Autodesk Inventor part; units mm, degrees
ref_plane "YZ Plane" through (0, 0, 0) normal (1, 0, 0) x (0, 1, 0)
ref_plane "XZ Plane" through (0, 0, 0) normal (0, 1, 0) x (-1, 0, 0)
ref_plane "XY Plane" through (0, 0, 0) normal (0, 0, 1) x (1, 0, 0)
sketch "草图1" plane through (0, 0, 0) normal (0, 0, 1) x (1, 0, 0)
  circle A0 centre (0, 0) radius 2.5
  dimension "d0" = 5
extrude "拉伸1" add sketch "草图1" along normal blind 3
sketch "草图2" plane through (0, 0, 3) normal (0, 0, 1) x (1, 0, 0)
  line L0 (-0.75, 2.5) -> (0.75, 2.5)
  line L1 (0.75, 2.5) -> (0.75, -2.5)
  line L2 (0.75, -2.5) -> (-0.75, -2.5)
  line L3 (-0.75, -2.5) -> (-0.75, 2.5)
  circle A0 centre (0, 0) radius 2.5
  point P0 (0, 2.5)
  dimension "d3" = 1.5
extrude "拉伸2" cut sketch "草图2" against normal blind 1.5 contours L0 A0 L3 | L0 L1 A0 | A0 L1 L3 | A0 L2 L3 | L1 L2 A0
sketch "草图3" plane through (0, 0, 0) normal (0, 0, -1) x (-1, 0, 0)
  circle A0 centre (0, 0) radius 1.5
  dimension "d6" = 3
extrude "拉伸3" add sketch "草图3" along normal blind 10
thread "螺纹1"
chamfer "倒角1" distance 0.2 angle 45 1 edges at (1.5, 0, -10)
properties part number "分离前导形片固定螺丝"
Work out the finished part from the listing and answer in its coordinate system (mm). A direction names the side the tool comes from. Give positions to 0.01 mm unless a question says otherwise; leave off trailing zeros. Loops run counter-clockwise (first coordinate to the right, second up) from the corner with the lowest first, then second, coordinate; pieces in that order, holes last. Notation, with made-up numbers: (25.25, -25.75) - (82.25, -25.75) arc R30 ccw to (82.25, 11.25) - close; hole circle Ø5 at (-38, -25.5). An arc over 180 degrees is marked (long way). Answer in a Markdown table with one row per item.
(1) Section C-C (z = 0.25) is taken. Give the vertices of the cut face in (x, y), and give its area (3 significant figures).
Results list:
| item | result |
|---|---|
| outline | circle Ø5 at (0, 0) |
| area | 19.6 mm² |
(2) Section D-D (y = -1.65) is taken. Give the vertices of the cut face in (x, z).
Results list:
| item | result |
|---|---|
| outline | (-1.88, 0) - (1.88, 0) - (1.88, 3) - (0.75, 3) - (0.75, 1.5) - (-0.75, 1.5) - (-0.75, 3) - (-1.88, 3) - close |
(3) Consider L1, parallel to Z at x = 2.15, y = -0.9; L2, parallel to Y at x = 0, z = -1.5; L3, parallel to Z at x = -0.4, y = -1.85. Determine where each line is inside the solid, lowest interval first. Write a range as [from, to].
Results list:
| item | result |
|---|---|
| L1 | z = [0, 3] |
| L2 | y = [-1.5, 1.5] |
| L3 | z = [0, 1.5] |
(4) For a pull along X with two mould halves and no side action, classify faces 4 (the face through (1.5, -0.07, -4.83)), 5 (the face through (0, 0, -10)), 6 (the face through (-0.75, 0, 2)) as pulls with the +X half, pulls with the -X half, needs draft (parallel to the pull), parting line crosses it, or undercut.
Results list:
| item | result |
|---|---|
| face 4 | parting line crosses it |
| face 5 | needs draft |
| face 6 | undercut |
(5) Flat-ended cylindrical pins translate along their axes: pin 1 Ø1.5 at (y, z) = (0, -1) entering from -X; pin 2 Ø1.5 at (y, z) = (1.5, -2.5) entering from -X; pin 3 Ø0.5 at (x, y) = (0, 1) entering from +Z. Find the tip coordinate at first contact, or state that the pin passes through.
Results list:
| item | result |
|---|---|
| pin 1 | stops at x = -1.5 |
| pin 2 | stops at x = -1.3 |
| pin 3 | stops at z = 1.5 |
(6) Section A-A (y = 0) is taken. Give the vertices of the cut face in (x, z).
Results list:
| item | result |
|---|---|
| outline | (-2.5, 0) - (-1.5, 0) - (-1.5, -9.8) - (-1.3, -10) - (1.3, -10) - (1.5, -9.8) - (1.5, 0) - (2.5, 0) - (2.5, 3) - (0.75, 3) - (0.75, 1.5) - (-0.75, 1.5) - (-0.75, 3) - (-2.5, 3) - close |
(7) Section B-B (x = 0) is taken. Give the vertices of the cut face in (y, z), and give its area (3 significant figures).
Results list:
| item | result |
|---|---|
| outline | (-2.5, 0) - (-1.5, 0) - (-1.5, -9.8) - (-1.3, -10) - (1.3, -10) - (1.5, -9.8) - (1.5, 0) - (2.5, 0) - (2.5, 1.5) - (-2.5, 1.5) - close |
| area | 37.5 mm² |
(8) A tool of negligible diameter and unlimited length cuts with its end or side. For faces 1 (the face through (0.75, 0, 2)), 2 (the face through (2, 0, 0)), 3 (the face through (-1, 0, 3)), from which of +Z, -Z, +X, -X, +Y, -Y can it reach the whole face along a straight path? Write none if from no direction.
Results list:
| item | result |
|---|---|
| face 1 | +Z, +Y, -Y |
| face 2 | -Z |
| face 3 | +Z, +X, -X, +Y, -Y |
